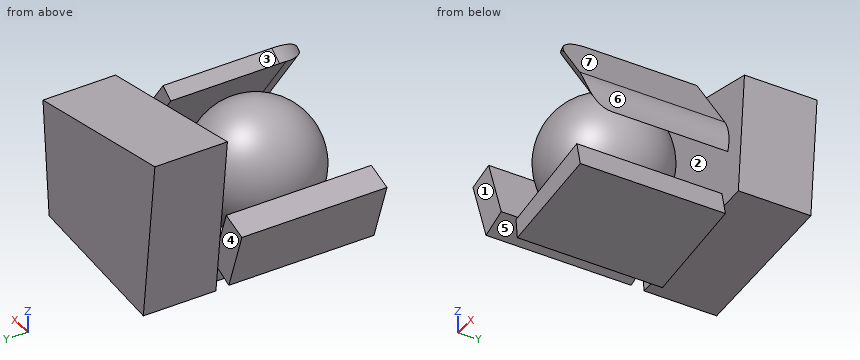
from build123d import *

# Parameters (mm, degrees)
BOSS_EXTRUDE1_START = -100
BOSS_EXTRUDE1_DEPTH = 200
BOSS_EXTRUDE2_START = 100
BOSS_EXTRUDE2_DEPTH = 100
FILLET4_R           = 50
FILLET5_R           = 50


with BuildPart() as part:
    # Sketch2 → Revolve1 (revolve)
    with BuildSketch(Plane.XY):
        with BuildLine():
            Line((0, 83.99866675223616), (0, -83.99866675223616))
            ThreePointArc((0, -83.99866675223616), (-83.99866675223616, 1.029e-14), (0, 83.99866675223616))
        make_face()
    revolve(axis=Axis((0, 83.99866675223616, 0), (0, -1, 0)))

    # Sketch3 → Cut-Revolve1 (revolve, cut)
    with BuildSketch(Plane.XY):
        with BuildLine():
            Line((0, 80.78753047196574), (0, -80.78753047196574))
            ThreePointArc((0, -80.78753047196574), (-80.78753047196574, 9.89e-15), (0, 80.78753047196574))
        make_face()
    revolve(axis=Axis((0, 80.78753047196574, 0), (0, -1, 0)), mode=Mode.SUBTRACT)

    # Sketch4 → Boss-Extrude1 (add)
    with BuildSketch(Plane(origin=(0, 0, 0), x_dir=(1, 0, 0), z_dir=(0, 1, 0)).offset(BOSS_EXTRUDE1_START)):
        Polygon((112.54766400764188, 11.102674962916051), (27.984824564062315, -106.46400649371546), (44.86622080796269, -118.60638205853901), (131.25655362126273, 1.5010410793763536), align=None)
        Polygon((-33.76429920229263, 94.6008743415586), (99.61989179054804, 62.66167239344396), (107.26781928097456, 94.6008743415586), (-30.8745618831775, 121.36896740283562), align=None)
        Polygon((-66.15977546395177, 65.39931827471092), (-93.84041715231778, -14.600778033423827), (-128.15679158223395, -2.7270515196505585), (-99.54190589937616, 79.97311259674068), align=None)
    extrude(amount=BOSS_EXTRUDE1_DEPTH)


with BuildPart() as boss_extrude1_piece_1:
    # of the separate pieces the step leaves, piece 1, a body of its own (boss_extrude1_pieces)
    add(part.part.solids().sort_by_distance((0, -83.998666752, 0))[0])



with BuildPart() as boss_extrude1_piece_2:
    # of the separate pieces the step leaves, piece 2, a body of its own (boss_extrude1_pieces)
    add(part.part.solids().sort_by_distance((-33.764299202, -100, -94.600874342))[0])


with BuildPart() as boss_extrude1_piece_3:
    # of the separate pieces the step leaves, piece 3, a body of its own (boss_extrude1_pieces)
    add(part.part.solids().sort_by_distance((112.547664008, -100, -11.102674963))[0])


with BuildPart() as boss_extrude1_piece_1_1:
    add(boss_extrude1_piece_1.part)

    add(boss_extrude1_piece_2.part)  # Boss-Extrude2 merges Boss-Extrude1 piece 2

    add(boss_extrude1_piece_3.part)  # Boss-Extrude2 merges Boss-Extrude1 piece 3
    # Sketch4<3> → Boss-Extrude2 (add)
    with BuildSketch(Plane(origin=(0, 0, 0), x_dir=(1, 0, 0), z_dir=(0, 1, 0)).offset(BOSS_EXTRUDE2_START)):
        Polygon((-71.1192338079553, 103.5456135287754), (-96.42597159573657, -118.60638205853901), (149.04960909120163, -75.4373531726898), (135.6655625605631, 78.63127336750127), align=None)
    extrude(amount=BOSS_EXTRUDE2_DEPTH)

    # Fillet4
    # the kernel refuses this fillet: 50 mm, written as the material it takes off along each edge
    with BuildSketch(Plane(origin=(-73.49181604435654, -100, 33.47434002763414), x_dir=(2e-16, 1, -2.8e-16), z_dir=(0.8118131248673509, 0, 0.5839173317286507))) as fillet4_piece_1:
        with BuildLine():
            CenterArc((FILLET4_R, -FILLET4_R), FILLET4_R, 90.00000000000003, 89.99999999999997)
            Line((1.73e-14, -FILLET4_R), (-FILLET4_R * 0.02, -FILLET4_R))
            Line((-FILLET4_R * 0.02, -FILLET4_R), (-FILLET4_R * 0.02, FILLET4_R * 0.02))
            Line((-FILLET4_R * 0.02, FILLET4_R * 0.02), (FILLET4_R, FILLET4_R * 0.02))
            Line((FILLET4_R, FILLET4_R * 0.02), (FILLET4_R, 0))
        make_face()
    extrude(amount=270.79468257754365, mode=Mode.SUBTRACT)
    with BuildSketch(Plane(origin=(171.7917074692354, -100, -93.46894402013166), x_dir=(0, 1, 0), z_dir=(-0.5839173317286501, 0, 0.8118131248673512))) as fillet4_piece_2:
        with BuildLine():
            CenterArc((40.583856818365355, -50), FILLET4_R, 90, 54.26011731322143)
            Line((0, -20.794682577543853), (-0.8116771363673081, -20.21057622909473))
            ThreePointArc((-0.8116771363673081, -20.21057622909473), (-1, -10.397341288771914), (-1, -6.48e-15))
            Line((-1, -6.48e-15), (0, 1.0000000000000047))
            Line((0, 1.0000000000000047), (40.583856818365355, 0.9999999999999881))
            Line((40.583856818365355, 0.9999999999999881), (40.583856818365355, 0))
        make_face()
    extrude(amount=347.739166716712, mode=Mode.SUBTRACT)

    # Fillet5
    # the kernel refuses this fillet: 50 mm, written as the material it takes off along each edge
    with BuildSketch(Plane(origin=(131.25655362126273, -209.28392328582004, -1.50104107937635), x_dir=(-0.8896758585741418, 0, -0.4565926704080605), z_dir=(0, 1, 0))) as fillet5_piece_1:
        with BuildLine():
            CenterArc((55.94900253333829, 35.785265930590285), FILLET5_R, 171.4409151223373, 54.26011731322126)
            Line((6.5058569003557185, 43.22672747491594), (5.516993987696065, 43.37555670580245))
            Line((5.516993987696065, 43.37555670580245), (-0.9888629126596437, 0.1488292308865173))
            Line((-0.9888629126596437, 0.1488292308865173), (-9.07e-15, -1.0000000000000053))
            ThreePointArc((-9.07e-15, -1.0000000000000053), (10.514441542566455, -0.9999999999999917), (20.330480696168753, -0.7157053186118065))
            Line((20.330480696168753, -0.7157053186118065), (21.02888308513286, 9.6e-16))
        make_face()
    extrude(amount=309.28392328582004, mode=Mode.SUBTRACT)


solid = boss_extrude1_piece_1_1.part
Geometry check sheet. Reference: the model listing, model coordinates, mm. Face numbers are marked on the shaded views. A direction names the side the tool comes from. Give positions to 0.01 mm unless a question says otherwise; leave off trailing zeros. Loops run counter-clockwise (first coordinate to the right, second up) from the corner with the lowest first, then second, coordinate; pieces in that order, holes last.
(1) Section check B-B on y = -66. Record the cut outline in (x, z), then the cut area to 3 significant figures.
From the geometry:
outline: (-128.16, 2.73) - (-99.54, -79.97) - (-66.16, -65.4) - (-93.84, 14.6) - close; circle Ø103.92 at (0, 0); (-33.76, -94.6) - (-30.87, -121.37) - (107.27, -94.6) - (99.62, -62.66) - close; (29.87, 104.58) - (112.72, -10.59) arc R50 ccw to (105.73, 33.99) - (46.4, 116.47) - close; hole circle Ø93.18 at (0, 0)
area: 11,600 mm2
(2) Section check D-D on y = 37. Record the cut outline in (x, z).
From the geometry:
outline: (-128.16, 2.73) - (-99.54, -79.97) - (-66.16, -65.4) - (-93.84, 14.6) - close; circle Ø150.82 at (0, 0); (-33.76, -94.6) - (-30.87, -121.37) - (107.27, -94.6) - (99.62, -62.66) - close; (27.98, 106.46) - (112.55, -11.1) arc R50 ccw to (105.73, 33.99) - (44.87, 118.61) - close; hole circle Ø143.63 at (0, 0)
(3) Section check A-A on x = -15. Record the cut outline in (y, z).
From the geometry:
outline: (-100, -118.29) - (100, -118.29) - (100, -96.78) - (200, -96.78) - (200, 104.29) - (100, 104.29) - (100, -90.11) - (-100, -90.11) - close; circle Ø165.3 at (0, 0); hole circle Ø158.77 at (0, 0)
(4) Thickness scan on L1, parallel to X at y = 1.5, z = 50.5; L2, parallel to X at y = -54.5, z = -33.5; L3, parallel to Y at x = -21.5, z = -84. Record the ranges inside material, lowest first.
From the geometry:
L1: x = -67.11 to -63.04, 63.04 to 67.11, 68.24 to 93.85
L2: x = -115.62 to -77.2, -54.44 to -49.34, 49.34 to 54.44
L3: y = 100 to 200
(5) Release check for a two-part mould opening along Y. For the marked faces 1, 2 and 3 record: released by +Y, released by -Y, zero draft, split by the parting line, or undercut.
From the geometry:
face 1: released by -Y
face 2: undercut
face 3: zero draft
(6) Section check C-C on x = -89. Record the cut outline in (y, z), then the cut area to 3 significant figures.
From the geometry:
outline: (-100, -75.37) - (100, -75.37) - (100, 0.61) - (-100, 0.61) - close; (100, 53.42) - (200, 53.42) - (200, 117.3) - (100, 117.3) - close
area: 21,600 mm2
(7) Set-up check for the marked faces 4, 5, 6 and 7: record each of +Z, -Z, +X, -X, +Y, -Y from which the full face is reachable in a straight line by a thin tool's end or side.
From the geometry:
face 4: -Z, -X, +Y
face 5: -Z, -Y
face 6: +X, -Y
face 7: +Z, +X, -Y
(8) Depth check by flat-ended pin: pin 1 Ø23 at (x, z) = (52, 109) entering from +Y; pin 2 Ø1 at (x, y) = (95.5, 133.5) entering from -Z; pin 3 Ø4 at (x, y) = (-67, 3.5) entering from +Z; pin 4 Ø2 at (x, y) = (116.5, 75) entering from -Z. Enter the tip coordinate at first touch or a pass-through.
From the geometry:
pin 1: stops at y = 100
pin 2: stops at z = -83.53
pin 3: stops at z = 53.09
pin 4: passes through
